Build history of the part. All positions in model axes, mm. Face numbers are marked on the shaded views. A direction names the side the tool comes from. Round coordinates to 2 decimals unless told otherwise and drop trailing zeros. Loops run counter-clockwise (first coordinate to the right, second up) from the corner with the lowest first, then second, coordinate; pieces in that order, holes last. Notation, with made-up numbers: (61, -11.75) - (120, -11.75) arc R16 cw to (120, -6.75) - close; hole circle Ø9 at (-28.5, 69). An arc over 180 degrees is marked (long way). Put each result on its own line as item: value. Start each with the question number.
Autodesk Inventor part; units mm, degrees
ref_plane "YZ Plane" through (0, 0, 0) normal (1, 0, 0) x (0, 1, 0)
ref_plane "XZ Plane" through (0, 0, 0) normal (0, 1, 0) x (-1, 0, 0)
ref_plane "XY Plane" through (0, 0, 0) normal (0, 0, 1) x (1, 0, 0)
sketch "Sketch1" plane through (0, 0, 0) normal (0, 0, 1) x (1, 0, 0)
  point P0 (0, 0)
sketch "Sketch2" plane through (0, 0, 0) normal (0, 0, 1) x (1, 0, 0)
  line L0 (-25, 25) -> (25, 25)
  line L1 (25, 25) -> (25, -25)
  line L2 (25, -25) -> (-25, -25)
  line L3 (-25, -25) -> (-25, 25)
  point P0 (0, 0)
  dimension "d0" = 50
  dimension "d1" = 50
  dimension "d2" = 25
  dimension "d3" = 25
extrude "Extrusion1" add sketch "Sketch2" along normal blind 38
sketch "Sketch3" plane through (0, 0, 0) normal (0, 0, -1) x (-1, 0, 0)
  point P0 (0, 0)
sketch "Sketch4" plane through (-25, 25, 0) normal (0, 1, 0) x (1, 0, 0)
  line L0 (0, 0) -> (50, 0)
  line L1 (46.25, 0) -> (3.75, 0)
  line L2 (3.75, 0) -> (3.75, -16)
  line L3 (3.75, -16) -> (46.25, -16)
  line L4 (46.25, -16) -> (46.25, 0)
  line L5 (50, 0) -> (50, -38)
  point P0 (25, 0)
  dimension "d6" = 42.5
  dimension "d7" = 16
  dimension "d8" = 3.75
extrude "Extrusion2" cut sketch "Sketch4" against normal blind 46.25
sketch "Sketch5" plane through (21.25, 25, 16) normal (0, 0, -1) x (-1, 0, 0)
  line L0 (0, -46.25) -> (0, 0)
  line L1 (42.5, 0) -> (42.5, -46.25)
  line L2 (0, -3.75) -> (42.5, -3.75)
  line L3 (42.5, -3.75) -> (42.5, -46.25)
  line L4 (42.5, -46.25) -> (0, -46.25)
  line L5 (0, -46.25) -> (0, -3.75)
  line L6 (-3.75, 0) -> (46.25, 0)
  point P0 (21.25, -25)
  dimension "d11" = 3.75
extrude "Extrusion3" cut sketch "Sketch5" against normal blind 18 contours L0 L2 L1 L4
sketch "Sketch6" plane through (-25, -25, 0) normal (-1, 0, 0) x (0, 0, 1)
  point P0 (0, 25)
sketch "Sketch7" plane through (0, 0, 38) normal (0, 0, 1) x (1, 0, 0)
  circle A0 centre (0, 0) radius 11.25
  dimension "d14" = 22.5
extrude "Extrusion4" cut sketch "Sketch7" against normal blind 6
sketch "Sketch8" plane through (0, 0, 38) normal (0, 0, 1) x (1, 0, 0)
  circle A0 centre (-14.5105, 15.5) radius 1.625
  circle A1 centre (16.4895, 15.5) radius 1.625
  circle A2 centre (15.5, -15.5) radius 1.625
  circle A3 centre (-15.5, -15.5) radius 1.625
  point P0 (0, 0)
  dimension "d17" = 3.25
  dimension "d18" = 3.25
  dimension "d19" = 3.25
  dimension "d20" = 3.25
  dimension "d21" = 15.5
  dimension "d22" = 31
  dimension "d23" = 31
  dimension "d24" = 15.5
  dimension "d25" = 31
  dimension "d26" = 15.5
  dimension "d27" = 15.5
extrude "Extrusion5" cut sketch "Sketch8" against normal blind 4
sketch "Sketch9" plane through (-25, -21.25, 0) normal (0, 1, 0) x (1, 0, 0)
  point P0 (25, 0)
sketch "Sketch10" plane through (-25, -25, 0) normal (0, -1, 0) x (1, 0, 0)
  line L0 (37.5, 6.9021) -> (37.5, 27.0979) construction
  line L1 (46.25, 34) -> (3.75, 34)
  line L2 (39.125, 6.9021) -> (39.125, 27.0979)
  line L3 (35.875, 27.0979) -> (35.875, 6.9021)
  arc A0 (35.875, 6.9021) -> (39.125, 6.9021) centre (37.5, 6.9021) ccw
  arc A1 (39.125, 27.0979) -> (35.875, 27.0979) centre (37.5, 27.0979) ccw
  line L4 (12.5, 6.9021) -> (12.5, 27.0979) construction
  line L5 (14.125, 6.9021) -> (14.125, 27.0979)
  line L6 (10.875, 27.0979) -> (10.875, 6.9021)
  arc A2 (10.875, 6.9021) -> (14.125, 6.9021) centre (12.5, 6.9021) ccw
  arc A3 (14.125, 27.0979) -> (10.875, 27.0979) centre (12.5, 27.0979) ccw
  line L7 (50, 0) -> (0, 0)
  line L8 (0, 0) -> (0, 38)
  point P0 (25, 0)
  point P1 (37.5, 17)
  point P2 (12.5, 17)
  dimension "d30" = 3.25
  dimension "d31" = 3.25
  dimension "d32" = 17
  dimension "d33" = 17
  dimension "d34" = 25
  dimension "d35" = 12.5
extrude "Extrusion6" cut sketch "Sketch10" against normal blind 4
sketch "Sketch11" plane through (0, 0, 38) normal (0, 0, 1) x (1, 0, 0)
  point P0 (0, 0)
sketch "Sketch12" plane through (0, 0, 38) normal (0, 0, 1) x (1, 0, 0)
  circle A0 centre (-14.5105, 15.5) radius 1.625
  circle A1 centre (-14.5105, 15.5) radius 3
  circle A2 centre (16.4895, 15.5) radius 1.625
  circle A3 centre (16.4895, 15.5) radius 3
  circle A4 centre (-15.5, -15.5) radius 1.625
  circle A5 centre (-15.5, -15.5) radius 3
  circle A6 centre (15.5, -15.5) radius 1.625
  circle A7 centre (15.5, -15.5) radius 3
  point P0 (0, 0)
  dimension "d38" = 6
  dimension "d39" = 6
  dimension "d40" = 6
  dimension "d41" = 6
extrude "Extrusion7" cut sketch "Sketch12" against normal blind 2
sketch "Sketch13" plane through (-25, -21.25, 0) normal (0, 1, 0) x (1, 0, 0)
  arc A0 (10.875, -27.0979) -> (14.125, -27.0979) centre (12.5, -27.0979) ccw
  arc A1 (14.125, -6.9021) -> (10.875, -6.9021) centre (12.5, -6.9021) ccw
  line L0 (12.5, -27.0979) -> (12.5, -6.9021) construction
  line L1 (15.5, -27.0979) -> (15.5, -6.9021)
  line L2 (9.5, -6.9021) -> (9.5, -27.0979)
  arc A2 (9.5, -27.0979) -> (15.5, -27.0979) centre (12.5, -27.0979) ccw
  arc A3 (15.5, -6.9021) -> (9.5, -6.9021) centre (12.5, -6.9021) ccw
  arc A4 (35.875, -27.0979) -> (39.125, -27.0979) centre (37.5, -27.0979) ccw
  arc A5 (39.125, -6.9021) -> (35.875, -6.9021) centre (37.5, -6.9021) ccw
  line L3 (37.5, -27.0979) -> (37.5, -6.9021) construction
  line L4 (40.5, -27.0979) -> (40.5, -6.9021)
  line L5 (34.5, -6.9021) -> (34.5, -27.0979)
  arc A6 (34.5, -27.0979) -> (40.5, -27.0979) centre (37.5, -27.0979) ccw
  arc A7 (40.5, -6.9021) -> (34.5, -6.9021) centre (37.5, -6.9021) ccw
  point P0 (25, 0)
  point P1 (12.5, -17)
  point P2 (37.5, -17)
  dimension "d44" = 6
  dimension "d45" = 6
extrude "Extrusion8" cut sketch "Sketch13" against normal blind 2
sketch "Sketch14" plane through (0, 0, 38) normal (0, 0, 1) x (1, 0, 0)
  line L0 (0, 0) -> (0, -25)
  line L1 (25, -25) -> (-25, -25)
properties part number "stepperMount"
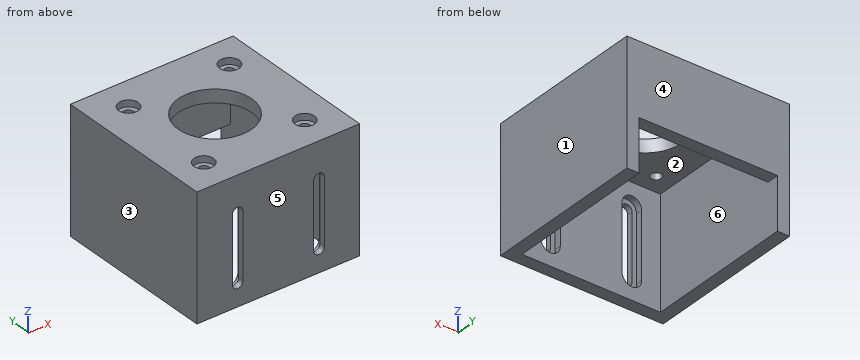
1) Slice it at B-B, the plane z = 31. Write the cut outline in (x, y), and give its area (3 significant figures).
2) Pull direction X, two halves, no side cores. Call the marked faces 1, 2, 3 and 4: pulls with the +X half, pulls with the -X half, needs draft (parallel to the pull), parting line crosses it, or undercut.
3) Slice it at C-C, the plane x = -2.5. Write the cut outline in (y, z).
4) Slice it at D-D, the plane z = 19. Write the cut outline in (x, y) (3 decimals), and give its area (3 significant figures).
5) Which spindle directions (+Z, -Z, +X, -X, +Y, -Y) get a long thin tool onto all of the face, cutting with end or side? Do the marked faces 5 and 6. Say none if no direction does.
6) Slice it at A-A, the plane y = 0. Write the cut outline in (x, z).
7) Drill centre lines: line 1 (Y direction, x = 16.5, z = 32); line 2 (Z direction, x = -13.5, y = 13). Where is each one in solid material? Low to high. Write a range as [from, to].
8) Drop flat-ended pins along their axis: pin 1 Ø10 at (x, y) = (-13.5, -8) entering from -Z; pin 2 Ø1.8 at (x, y) = (-14, -15) entering from +Z; pin 3 Ø1.8 at (x, z) = (12, 12.5) entering from +Y; pin 4 Ø1 at (x, z) = (-15.5, 15) entering from +Y. Give the stop position or say it passes through.
Taken from the geometry:
1. outline: (-25, -25) - (25, -25) - (25, 25) - (-25, 25) - close; hole (-21.25, -21.25) - (21.25, -21.25) - (21.25, 21.25) - (-21.25, 21.25) - close
1. area: 694 mm2
2. face 1: pulls with the +X half
2. face 2: undercut
2. face 3: pulls with the -X half
2. face 4: needs draft
3. outline: (-25, 0) - (-21.25, 0) - (-21.25, 34) - (-10.97, 34) - (-10.97, 38) - (-25, 38) - close; (10.97, 34) - (21.25, 34) - (21.25, 16) - (25, 16) - (25, 38) - (10.97, 38) - close
4. outline: (-25, -25) - (-14.125, -25) - (-14.125, -23.25) - (-15.5, -23.25) - (-15.5, -21.25) - (-21.25, -21.25) - (-21.25, 21.25) - (21.25, 21.25) - (21.25, -21.25) - (15.5, -21.25) - (15.5, -23.25) - (14.125, -23.25) - (14.125, -25) - (25, -25) - (25, 25) - (-25, 25) - close; (-10.875, -25) - (10.875, -25) - (10.875, -23.25) - (9.5, -23.25) - (9.5, -21.25) - (-9.5, -21.25) - (-9.5, -23.25) - (-10.875, -23.25) - close
4. area: 658 mm2
5. face 5: +Z, -Z, +X, -X, -Y
5. face 6: -Z
6. outline: (-25, 0) - (-21.25, 0) - (-21.25, 34) - (-11.25, 34) - (-11.25, 38) - (-25, 38) - close; (11.25, 34) - (21.25, 34) - (21.25, 0) - (25, 0) - (25, 38) - (11.25, 38) - close
7. line 1: y = [-25, -21.25], [21.25, 25]
7. line 2: z = [34, 36]
8. pin 1: stops at z = 34
8. pin 2: stops at z = 36
8. pin 3: passes through
8. pin 4: stops at y = -21.25
